Source: CAD feature listing. Evaluate the final solid. Frame: model axes, mm. Face numbers are marked on the shaded views. A direction names the side the tool comes from. Give positions to 0.01 mm unless a question says otherwise; leave off trailing zeros. Write each loop counter-clockwise with the first axis right and the second up, starting at its lowest first coordinate (ties: lowest second). Pieces come first, ordered by that corner, then holes. Notation, with made-up numbers: (1, 78) -> (26, 78) arc R17 ccw to (26, 85) -> close; hole circle Ø4 at (86.5, 24). An arc over 180 degrees is marked (long way). Answer as a JSON object with one key per item and string values. Group by question number.
Item 1: Section query D-D on y = 19. Return the cut outline in (x, z).
Item 2: Ray query, probe 1 along Y at (x, z) = (5.08, -6.45); probe 2 along Y at (x, z) = (9.75, -2.75); probe 3 along X at (y, z) = (22.5, -1). Return the intervals inside material, ascending. Write a range as from..to.
Item 3: Section query B-B on x = 5.08. Return the cut outline in (y, z).
Item 4: Section query C-C on x = 7. Return the cut outline in (y, z), plus the area to 3 significant figures.
Item 5: First-contact query: pin 1 Ø1 at (y, z) = (7, -6) entering from -X; pin 2 Ø0.8 at (x, z) = (5.5, -4) entering from -Y; pin 3 Ø1.3 at (x, z) = (6.5, -3.5) entering from +Y. Flat tips, straight axial feed; report the tip coordinate or a pass-through.
Item 6: Section query A-A on y = 5. Return the cut outline in (x, z).
Item 7: Access query for the marked faces 1, 2 and 3. Directions: +Z, -Z, +X, -X, +Y, -Y. A direction counts if a zero-diameter tool reaches every point of the face in a straight line with its end or side. Return the directions, or none.
Item 8: Pull-direction query (Z, two-part tool) for the marked faces 4, 5 and 6; classes: pulls with the +Z half, pulls with the -Z half, needs draft (parallel to the pull), parting line crosses it, or undercut.
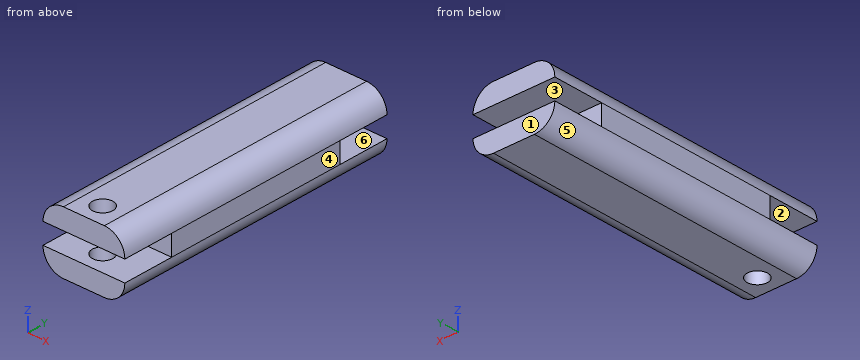
from build123d import *

# Parameters (mm, degrees)
SKETCH1_W               = 10.16
SKETCH1_H               = 7.62
BOSS_EXTRUDE1_DEPTH     = 35.56
FILLET1_R               = 2.54
SKETCH2_W               = 10.16
SKETCH2_H               = 2.54
CUT_EXTRUDE1_DEPTH      = 6.35
CUT_EXTRUDE2_DEPTH      = 38.759814618
CUT_EXTRUDE2_DEPTH_BACK = 38.759814618
SKETCH3_R               = 1.27


with BuildPart() as part:
    # Sketch1 → Boss-Extrude1 (new body)
    with BuildSketch(Plane(origin=(0, 0, 0), x_dir=(1, 0, 0), z_dir=(0, 1, 0))):
        with Locations((5.08, 3.81)):
            Rectangle(SKETCH1_W, SKETCH1_H)
    extrude(amount=BOSS_EXTRUDE1_DEPTH)

    # Fillet1
    fillet1_edges = [part.edges().sort_by_distance(p)[0] for p in [
        (0, 17.78, -7.62),
        (10.16, 17.78, -7.62),
        (10.16, 17.78, 0),
        (0, 17.78, 0),
    ]]
    fillet(fillet1_edges, radius=FILLET1_R)

    # Sketch2 → Cut-Extrude1 (cut)
    with BuildSketch(Plane(origin=(0, 0, 0), x_dir=(1, 0, 0), z_dir=(0, 1, 0))):
        with Locations((5.08, 3.81)):
            Rectangle(SKETCH2_W, SKETCH2_H)
    cut_extrude1 = extrude(amount=CUT_EXTRUDE1_DEPTH, mode=Mode.SUBTRACT)

    # Mirror1: Cut-Extrude1 across plane
    add(cut_extrude1.mirror(Plane.ZX.offset(17.78)), mode=Mode.SUBTRACT)

    # Sketch3 → Cut-Extrude2 (cut, two sides: drawn at the far end of the back side and taken through both)
    with BuildSketch(Plane.XY.offset(-CUT_EXTRUDE2_DEPTH_BACK)):
        with Locations(Location((5.08, 2.54, 0), (0, 0, 180))):
            Circle(SKETCH3_R)
    extrude(amount=CUT_EXTRUDE2_DEPTH + CUT_EXTRUDE2_DEPTH_BACK, mode=Mode.SUBTRACT)


solid = part.part
Worked answers:
{
 "1": {"outline": "(0, -5.08) arc R2.54 ccw to (2.54, -7.62) -> (7.62, -7.62) arc R2.54 ccw to (10.16, -5.08) -> (10.16, -2.54) arc R2.54 ccw to (7.62, 0) -> (2.54, 0) arc R2.54 ccw to (0, -2.54) -> close"},
 "2": {"probe 1": "0..1.27, 3.81..35.56", "probe 2": "6.35..29.21", "probe 3": "0.52..9.64"},
 "3": {"outline": "(0, -7.62) -> (1.27, -7.62) -> (1.27, -5.08) -> (0, -5.08) -> close; (0, -2.54) -> (1.27, -2.54) -> (1.27, 0) -> (0, 0) -> close; (3.81, -7.62) -> (35.56, -7.62) -> (35.56, -5.08) -> (29.21, -5.08) -> (29.21, -2.54) -> (35.56, -2.54) -> (35.56, 0) -> (3.81, 0) -> (3.81, -2.54) -> (6.35, -2.54) -> (6.35, -5.08) -> (3.81, -5.08) -> close"},
 "4": {"outline": "(0, -7.62) -> (35.56, -7.62) -> (35.56, -5.08) -> (29.21, -5.08) -> (29.21, -2.54) -> (35.56, -2.54) -> (35.56, 0) -> (0, 0) -> (0, -2.54) -> (6.35, -2.54) -> (6.35, -5.08) -> (0, -5.08) -> close", "area": "239 mm^2"},
 "5": {"pin 1": "x = 0.03", "pin 2": "y = 6.35", "pin 3": "y = 29.21"},
 "6": {"outline": "(0, -5.08) arc R2.54 ccw to (2.54, -7.62) -> (7.62, -7.62) arc R2.54 ccw to (10.16, -5.08) -> close; (0, -2.54) -> (10.16, -2.54) arc R2.54 ccw to (7.62, 0) -> (2.54, 0) arc R2.54 ccw to start"},
 "7": {"face 1": "+Z, -Z, +X, -X, +Y", "face 2": "+X, -X, -Y", "face 3": "+X, -X, +Y"},
 "8": {"face 4": "needs draft", "face 5": "pulls with the -Z half", "face 6": "undercut"}
}
